```python
from build123d import *

# Parameters (mm, degrees)
SKETCH1_R           = 26.035
BOSS_EXTRUDE1_DEPTH = 10.16
SKETCH2_R           = 6.223
SKETCH2_R_2         = 3.429
SKETCH2_R_3         = 3.45
CUT_EXTRUDE1_DEPTH  = 39.195131234
SKETCH3_W           = 21.082
SKETCH3_H           = 18.542
CUT_EXTRUDE2_DEPTH  = 7.62


with BuildPart() as part:
    # Sketch1 → Boss-Extrude1 (new body)
    with BuildSketch(Plane(origin=(0, 0, 0), x_dir=(1, 0, 0), z_dir=(0, 1, 0))):
        with Locations(Location((0, 0, 0), (0, 0, 270))):
            Circle(SKETCH1_R)
    extrude(amount=BOSS_EXTRUDE1_DEPTH)

    # Sketch2 → Cut-Extrude1 (cut, through all)
    with BuildSketch(Plane(origin=(0, 10.16, 0), x_dir=(1, 0, 0), z_dir=(0, 1, 0))):
        with Locations(Location((0, 17.293004752, 0), (0, 0, 270))):
            Circle(SKETCH2_R)
        with Locations(Location((0, -20.598576002, 0), (0, 0, 270))):
            Circle(SKETCH2_R_2)
        with Locations(Location((0, 0, 0), (0, 0, 270))):
            Circle(SKETCH2_R_3)
    extrude(amount=-CUT_EXTRUDE1_DEPTH, mode=Mode.SUBTRACT)

    # Sketch3 → Cut-Extrude2 (cut)
    with BuildSketch(Plane.XZ):
        with Locations((0, 2.265)):
            Rectangle(SKETCH3_W, SKETCH3_H)
    extrude(amount=-CUT_EXTRUDE2_DEPTH, mode=Mode.SUBTRACT)


solid = part.part
```
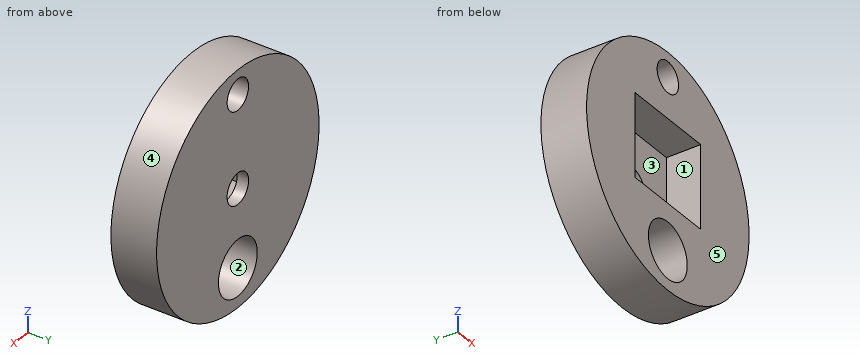
Geometry: final body of the model. Coordinates: model frame, mm. Face numbers are marked on the shaded views. A direction names the side the tool comes from. Give positions to 0.01 mm unless a question says otherwise; leave off trailing zeros. Write each loop counter-clockwise with the first axis right and the second up, starting at its lowest first coordinate (ties: lowest second). Pieces come first, ordered by that corner, then holes.
1. Section query A-A, the plane z = 0. Return loops of the section in (x, y) (3 decimals).
2. Pin query (flat end, axial travel): P1, Ø5.5, axis at x = -0.5, z = -1.5, coming from the -Y side; P2, Ø10, axis at x = 0, z = -17.29, coming from the +Y side; P3, Ø5, axis at y = 2, z = 0.5, coming from the +X side (3 decimals); P4, Ø1, axis at x = 2.5, y = 2, coming from the -Z side. Return the tip coordinate at first contact, or that it passes through.
3. Section query D-D, the plane z = -15. Return loops of the section in (x, y).
4. Section query B-B, the plane x = 0. Return loops of the section in (y, z) (3 decimals).
5. Draft query along X for the marked faces 3, 4 and 5. Return one class per face: released by +X, released by -X, zero draft, split by the parting line, or undercut.
6. Section query C-C, the plane y = 1.5. Return loops of the section in (x, z) (3 decimals), then the cut area to 3 significant figures.
7. Line query: probe 1 along Z at (x, y) = (1.5, 4); probe 2 along X at (y, z) = (6.25, 7); probe 3 along Z at (x, y) = (-8, 2). Output: solid intervals per line, ascending.
8. Reachability of the marked faces 1 and 2 from +Z, -Z, +X, -X, +Y, -Y: full face, straight path, thin tool, end or side. Return the list, or none.
Computed:
1. outline: (-26.035, 0) - (-10.541, 0) - (-10.541, 7.62) - (-3.45, 7.62) - (-3.45, 10.16) - (-26.035, 10.16) - close; (3.45, 7.62) - (10.541, 7.62) - (10.541, 0) - (26.035, 0) - (26.035, 10.16) - (3.45, 10.16) - close
2. P1: stops at y = 7.62
2. P2: passes through
2. P3: stops at x = 26.035
2. P4: stops at z = -25.96
3. outline: (-21.28, 0) - (-5.79, 0) - (-5.79, 10.16) - (-21.28, 10.16) - close; (5.79, 0) - (21.28, 0) - (21.28, 10.16) - (5.79, 10.16) - close
4. outline: (0, -26.035) - (10.16, -26.035) - (10.16, -23.516) - (0, -23.516) - close; (0, -11.07) - (10.16, -11.07) - (10.16, -3.45) - (7.62, -3.45) - (7.62, -7.006) - (0, -7.006) - close; (0, 11.536) - (7.62, 11.536) - (7.62, 3.45) - (10.16, 3.45) - (10.16, 17.17) - (0, 17.17) - close; (0, 24.028) - (10.16, 24.028) - (10.16, 26.035) - (0, 26.035) - close
5. face 3: undercut
5. face 4: split by the parting line
5. face 5: zero draft
6. outline: circle Ø52.07 at (0, 0); hole (-10.541, -7.006) - (10.541, -7.006) - (10.541, 11.536) - (-10.541, 11.536) - close; hole circle Ø12.446 at (0, -17.293); hole circle Ø6.858 at (0, 20.599)
6. area: 1,580 mm2
7. probe 1: z = -25.99 to -23.33, -11.25 to -7.01, 11.54 to 17.52, 23.68 to 25.99
7. probe 2: x = -25.08 to -10.54, 10.54 to 25.08
7. probe 3: z = -24.78 to -7.01, 11.54 to 24.78
8. face 1: -Y
8. face 2: +Y, -Y
